Read the model definition and answer for the solid it produces. Units are mm, in the model's axes. A direction names the side the tool comes from. Coordinates: 2 decimals unless noted, no trailing zeros. One line per item, written item: value. Start each with the question number.
1. Consider probe 1 along X at (y, z) = (-7.5, -2.75); probe 2 along X at (y, z) = (-63, -4); probe 3 along Z at (x, y) = (-11, -59). Determine where each line is inside the solid, lowest interval first.
2. Determine the mould class of faces 1 (the face through (10.676, 1.4, -1.777)), 2 (the face through (0, 1, -1.702)), 3 (the face through (0, -100, -3)) for opening direction Z: +Z half, -Z half, draft (parallel to the pull), parting line (faces both ways), or undercut.
3. For faces 4 (the face through (8, 1, 6.35)), 5 (the face through (-5.46, 1.4, 0.81)), determine the directions among +Z, -Z, +X, -X, +Y, -Y from which every point of the face is accessible in a straight line to the end or side of a thin tool.
4. Flat-ended cylindrical pins translate along their axes: pin 1 (3.5 mm diameter, centred on x = 8, y = 32.5, fed in from +Z); pin 2 (1 mm diameter, centred on x = 0, y = -25, fed in from +Z); pin 3 (2.5 mm diameter, centred on x = -8.74, z = -2.39, fed in from -Y). Find the tip coordinate at first contact, or state that the pin passes through.
5. The part is cut by section A-A (y = -43.5). State how many separate pieces and enclosed holes the cut face has, then the cut area to 3 significant figures.
```python
from build123d import *

# Parameters (mm, degrees)
SKETCH18_R                = 2.032
F_10_1050_PROFILE_1_DEPTH = 200


with BuildPart() as part:
    # Sketch18 → 10 1050 PROFILE(1) (new body)
    with BuildSketch(Plane.XZ.offset(-100)):
        with BuildLine():
            Line((9.551093887, 6.35), (6.330982008, 6.35))
            ThreePointArc((6.330982008, 6.35), (5.824379679, 5.843397671), (5.31777735, 6.35))
            Line((5.31777735, 6.35), (4.28752, 6.35))
            ThreePointArc((4.28752, 6.35), (3.545750844, 6.042749156), (3.2385, 5.30098))
            Line((3.2385, 5.30098), (3.2385, 5.18922))
            ThreePointArc((3.2385, 5.18922), (3.545750844, 4.447450844), (4.28752, 4.1402))
            Line((4.28752, 4.1402), (6.541264932, 4.1402))
            ThreePointArc((6.541264932, 4.1402), (7.403778411, 3.563601238), (7.200674335, 2.54618079))
            Line((7.200674335, 2.54618079), (3.874487735, -0.773919123))
            ThreePointArc((3.874487735, -0.773919123), (2.845157282, -1.460673567), (1.631480681, -1.7018))
            Line((1.631480681, -1.7018), (-1.631480681, -1.7018))
            ThreePointArc((-1.631480681, -1.7018), (-2.845157282, -1.460673567), (-3.874487735, -0.773919123))
            Line((-3.874487735, -0.773919123), (-7.091634343, 2.437340333))
            ThreePointArc((-7.091634343, 2.437340333), (-7.30860647, 3.524230776), (-6.387200124, 4.1402))
            Line((-6.387200124, 4.1402), (-4.28752, 4.1402))
            ThreePointArc((-4.28752, 4.1402), (-3.545750844, 4.447450844), (-3.2385, 5.18922))
            Line((-3.2385, 5.18922), (-3.2385, 5.30098))
            ThreePointArc((-3.2385, 5.30098), (-3.545750844, 6.042749156), (-4.28752, 6.35))
            Line((-4.28752, 6.35), (-5.319235427, 6.35))
            ThreePointArc((-5.319235427, 6.35), (-5.825837756, 5.843397671), (-6.332440085, 6.35))
            Line((-6.332440085, 6.35), (-9.552501021, 6.35))
            ThreePointArc((-9.552501021, 6.35), (-10.056951984, 5.843402239), (-10.565687406, 6.345697309))
            Line((-10.565687406, 6.345697309), (-10.591304516, 6.345701455))
            ThreePointArc((-10.591304516, 6.345701455), (-12.082359481, 5.728298321), (-12.7, 4.237343309))
            Line((-12.7, 4.237343309), (-12.7, -4.233074923))
            ThreePointArc((-12.7, -4.233074923), (-12.072915167, -5.733409532), (-10.564685825, -6.341261141))
            ThreePointArc((-10.564685825, -6.341261141), (-10.053713904, -5.834598435), (-9.551557924, -6.35))
            Line((-9.551557924, -6.35), (-6.323021107, -6.35))
            ThreePointArc((-6.323021107, -6.35), (-5.816495529, -5.83457959), (-5.309969951, -6.35))
            Line((-5.309969951, -6.35), (5.309969951, -6.35))
            ThreePointArc((5.309969951, -6.35), (5.816495529, -5.83457959), (6.323021107, -6.35))
            Line((6.323021107, -6.35), (9.550160942, -6.35))
            ThreePointArc((9.550160942, -6.35), (10.051855758, -5.834602622), (10.563288148, -6.340338775))
            Line((10.563288148, -6.340338775), (10.589922543, -6.34049468))
            ThreePointArc((10.589922543, -6.34049468), (12.081868228, -5.723579066), (12.7, -4.23213684))
            Line((12.7, -4.23213684), (12.7, 4.244714967))
            ThreePointArc((12.7, 4.244714967), (12.082266163, 5.735759476), (10.591047766, 6.353073372))
            Line((10.591047766, 6.353073372), (10.564289268, 6.353065837))
            ThreePointArc((10.564289268, 6.353065837), (10.059229141, 5.84339999), (9.551093887, 6.35))
        make_face()
        with Locations((-8.7376, -2.3876)):
            Circle(SKETCH18_R, mode=Mode.SUBTRACT)
        with Locations((8.7376, -2.3876)):
            Circle(SKETCH18_R, mode=Mode.SUBTRACT)
    extrude(amount=F_10_1050_PROFILE_1_DEPTH)


solid = part.part
```
Answer block:
1. probe 1: x = -12.7 to -10.74, -6.74 to 6.74, 10.74 to 12.7
1. probe 2: x = -12.7 to -9.97, -7.5 to 7.5, 9.97 to 12.7
1. probe 3: z = -6.3 to 6.31
2. face 1: undercut
2. face 2: +Z half
2. face 3: draft
3. face 4: +Z, +X, -X, +Y, -Y
3. face 5: +Y, -Y
4. pin 1: stops at z = 6.35
4. pin 2: stops at z = -1.7
4. pin 3: passes through
5. separate pieces: 1
5. enclosed holes: 2
5. area: 208 mm2
